CAD build for the part. Positions are in the model's coordinates, mm. A direction names the side the tool comes from. Give positions to 0.01 mm unless a question says otherwise; leave off trailing zeros. Write each loop counter-clockwise with the first axis right and the second up, starting at its lowest first coordinate (ties: lowest second). Pieces come first, ordered by that corner, then holes. Notation, with made-up numbers: (4, 54.5) - (20, 54.5) arc R23 ccw to (20, 62.5) - close; hole circle Ø5 at (12, 1). An arc over 180 degrees is marked (long way). Put each result on its own line as item: value. Start each with the question number.
1. Drop a flat-ended pin along its axis: pin 1 (1 mm diameter, centred on x = 4.5, z = 15, fed in from -Y). Give the stop position or say it passes through.
2. Wall check: line 1 (X direction, y = -10, z = 5.5); line 2 (Z direction, x = 29, y = -16.75); line 3 (X direction, y = -1.75, z = 9). Give the ranges that are in metal, low to high.
3. Mould opens along X. For faces 3 (the flat face through (20, -2, 24)), 4 (the flat face through (20, 0, 24)), 5 (the cylindrical face through (-1.93, -0.6, 12.33)) say: +X half, -X half, draft (parallel to the pull), parting line (faces both ways), or undercut.
4. Tool access for faces 1 (the flat face through (16, -13, 24.8)), 2 (the flat face through (-2.5, -16, 12)): list every direction of +Z, -Z, +X, -X, +Y, -Y with a clear straight run to the whole face (end or side of a thin tool).
5. Cut at A-A on z = 12.15. List the corners of the cut face in (x, y), and give its area (3 significant figures).
6. Cut at B-B on x = 16.25. List the corners of the cut face in (y, z).
7. Cut at C-C on y = -6. List the corners of the cut face in (x, z), and give its area (3 significant figures).
8. Cut at D-D on y = -23. List the corners of the cut face in (x, z), and give its area (3 significant figures).
from build123d import *

# Parameters (mm, degrees)
F0_W     = 37.5
F0_H     = 29.3
F1_DEPTH = 30
F2_W     = 33.5
F2_H     = 25.3
F3_DEPTH = 28
F4_R     = 11.9
F5_DEPTH = 2.001
F7_DEPTH = 29.301
F8_R     = 2


with BuildPart() as f1:
    # F0 (on Front) → F1 (new body)
    with BuildSketch(Plane.XZ):
        with Locations((16.25, 12.15)):
            Rectangle(F0_W, F0_H)
    extrude(amount=F1_DEPTH)

    # F2 (on face) → F3 (cut)
    with BuildSketch(Plane.XZ.offset(30)):
        with Locations((16.25, 12.15)):
            Rectangle(F2_W, F2_H)
    extrude(amount=-F3_DEPTH, mode=Mode.SUBTRACT)

    # F4 (on face) → F5 (cut, through all)
    with BuildSketch(Plane.XZ.offset(2)):
        with Locations((16.25, 12.15)):
            Circle(F4_R)
    extrude(amount=-F5_DEPTH, mode=Mode.SUBTRACT)

    # F6 (on face) → F7 (cut, through all)
    with BuildSketch(Plane.XY.offset(26.8)):
        with BuildLine():
            Line((2.75, -30), (29.75, -30))
            ThreePointArc((29.75, -30), (16.25, -16.5), (2.75, -30))
        make_face()
    extrude(amount=-F7_DEPTH, mode=Mode.SUBTRACT)

    # F8
    f8_edges = [f1.edges().sort_by_distance(p)[0] for p in [
        (-2.5, -15, 26.8),
        (-2.5, -15, -2.5),
        (35, -15, -2.5),
        (35, -15, 26.8),
        (16.25, 0, 26.8),
        (35, 0, 12.15),
        (16.25, 0, -2.5),
        (-2.5, 0, 12.15),
    ]]
    fillet(f8_edges, radius=F8_R)


solid = f1.part
Report:
1. pin 1: stops at y = -2
2. line 1: x = -2.5 to -0.5, 33 to 35
2. line 2: z = -2.5 to -0.5, 24.8 to 26.8
2. line 3: x = -2.48 to 4.77, 27.73 to 34.98
3. face 3: undercut
3. face 4: draft
3. face 5: -X half
4. face 1: -Y
4. face 2: +Z, -Z, -X, +Y, -Y
5. outline: (-2.5, -30) - (-0.5, -30) - (-0.5, -2) - (4.35, -2) - (4.35, 0) - (-0.5, 0) arc R2 ccw to (-2.5, -2) - close; (28.15, -2) - (33, -2) - (33, -30) - (35, -30) - (35, -2) arc R2 ccw to (33, 0) - (28.15, 0) - close
5. area: 138 mm²
6. outline: (-16.5, -2.5) - (-2, -2.5) arc R2 ccw to (0, -0.5) - (0, 0.25) - (-2, 0.25) - (-2, -0.5) - (-16.5, -0.5) - close; (-16.5, 24.8) - (-2, 24.8) - (-2, 24.05) - (0, 24.05) - (0, 24.8) arc R2 ccw to (-2, 26.8) - (-16.5, 26.8) - close
7. outline: (-2.5, -0.5) arc R2 ccw to (-0.5, -2.5) - (33, -2.5) arc R2 ccw to (35, -0.5) - (35, 24.8) arc R2 ccw to (33, 26.8) - (-0.5, 26.8) arc R2 ccw to (-2.5, 24.8) - close; hole (-0.5, -0.5) - (33, -0.5) - (33, 24.8) - (-0.5, 24.8) - close
7. area: 248 mm²
8. outline: (-2.5, -0.5) arc R2 ccw to (-0.5, -2.5) - (4.71, -2.5) - (4.71, -0.5) - (-0.5, -0.5) - (-0.5, 24.8) - (4.71, 24.8) - (4.71, 26.8) - (-0.5, 26.8) arc R2 ccw to (-2.5, 24.8) - close; (27.79, -2.5) - (33, -2.5) arc R2 ccw to (35, -0.5) - (35, 24.8) arc R2 ccw to (33, 26.8) - (27.79, 26.8) - (27.79, 24.8) - (33, 24.8) - (33, -0.5) - (27.79, -0.5) - close
8. area: 155 mm²
